Read the model definition and answer for the solid it produces. Units are mm, in the model's axes. Give positions to 0.01 mm unless a question says otherwise; leave off trailing zeros. Loops run counter-clockwise (first coordinate to the right, second up) from the corner with the lowest first, then second, coordinate; pieces in that order, holes last.
(1) Find section D-D, the plane z = 103.5. Write down the section's boundary in (x, y), then the cut area to 3 significant figures.
(2) Straight lines are drawn through the part: probe 1 along Z at (x, y) = (32.5, -1.4); probe 2 along X at (y, z) = (-1.4, 33.5); probe 3 along X at (y, z) = (-1, 34). For each, find the intervals that lie inside material, in ascending order.
(3) Find section C-C, the plane y = -1.1. Write down the section's boundary in (x, z).
(4) This flat-tipped pin is pushed along its axis until it touches: P1, Ø9.5, axis at x = 59.5, z = 39, coming from the -Y side. Where does it stop, or does it pass through?
(5) Determine the mould class of faces 1 (the face through (53.79, -1.52, 44.24)), 2 (the face through (2.85, -1.48, 3.01)), 3 (the face through (147.15, -1.48, 176.99)) for opening direction X: pulls with the +X half, pulls with the -X half, needs draft (parallel to the pull), parting line crosses it, or undercut.
(6) Find section A-A, the plane x = 114. Write down the section's boundary in (y, z).
(7) Find section B-B, the plane z = 39. Write down the section's boundary in (x, y).
```python
from build123d import *

# Parameters (mm, degrees)
F1_DEPTH = 3
F2_W     = 103
F2_H     = 57
F3_DEPTH = 3.001
F4_R     = 7.75
F5_DEPTH = 25


with BuildPart() as f1:
    # F0 (on Front) → F1 (new body)
    with BuildSketch(Plane.XZ):
        with BuildLine():
            ThreePointArc((0, 10), (2.928932, 2.928932), (10, 0))
            Line((10, 0), (140, 0))
            ThreePointArc((140, 0), (147.071068, 2.928932), (150, 10))
            Line((150, 10), (150, 170))
            ThreePointArc((150, 170), (147.071068, 177.071068), (140, 180))
            Line((140, 180), (10, 180))
            ThreePointArc((10, 180), (2.928932, 177.071068), (0, 170))
            Line((0, 170), (0, 10))
        make_face()
    extrude(amount=F1_DEPTH)

    # F2 (on face) + F1_face (on face) → F3 (cut, through all)
    with BuildSketch(Plane.XZ):
        with Locations((75, 96.5)):
            Rectangle(F2_W, F2_H)
    with BuildSketch(Plane(origin=(75, -3, 90), x_dir=(1, 0, 0), z_dir=(0, -1, 0))):
        with BuildLine():
            Line((-75, 80), (-75, -80))
            ThreePointArc((-75, -80), (-72.071068, -87.071068), (-65, -90))
            Line((-65, -90), (65, -90))
            ThreePointArc((65, -90), (72.071068, -87.071068), (75, -80))
            Line((75, -80), (75, 80))
            ThreePointArc((75, 80), (72.071068, 87.071068), (65, 90))
            Line((65, 90), (-65, 90))
            ThreePointArc((-65, 90), (-72.071068, 87.071068), (-75, 80))
        make_face()
    extrude(amount=F3_DEPTH, mode=Mode.SUBTRACT)

    # F4 (on face) → F5 (cut)
    with BuildSketch(Plane.XZ.offset(3)):
        with Locations((32.5, 39)):
            Circle(F4_R)
        with Locations((59.5, 39)):
            Circle(F4_R)
    extrude(amount=-F5_DEPTH, mode=Mode.SUBTRACT)


solid = f1.part
```
Entries:
1. outline: (0, -3) - (23.5, -3) - (23.5, 0) - (0, 0) - close; (126.5, -3) - (150, -3) - (150, 0) - (126.5, 0) - close
1. area: 141 mm2
2. probe 1: z = 0 to 31.25, 46.75 to 68, 125 to 180
2. probe 2: x = 0 to 27.04, 37.96 to 54.04, 64.96 to 150
2. probe 3: x = 0 to 26.58, 38.42 to 53.58, 65.42 to 150
3. outline: (0, 10) arc R10 ccw to (10, 0) - (140, 0) arc R10 ccw to (150, 10) - (150, 170) arc R10 ccw to (140, 180) - (10, 180) arc R10 ccw to (0, 170) - close; hole (23.5, 68) - (126.5, 68) - (126.5, 125) - (23.5, 125) - close; hole circle Ø15.5 at (32.5, 39); hole circle Ø15.5 at (59.5, 39)
4. P1: passes through
5. face 1: undercut
5. face 2: pulls with the -X half
5. face 3: pulls with the +X half
6. outline: (-3, 0) - (0, 0) - (0, 68) - (-3, 68) - close; (-3, 125) - (0, 125) - (0, 180) - (-3, 180) - close
7. outline: (0, -3) - (24.75, -3) - (24.75, 0) - (0, 0) - close; (40.25, -3) - (51.75, -3) - (51.75, 0) - (40.25, 0) - close; (67.25, -3) - (150, -3) - (150, 0) - (67.25, 0) - close
